Geometry: final body of the model. Coordinates: model frame, mm. Face numbers are marked on the shaded views. A direction names the side the tool comes from. Coordinates: 2 decimals unless noted, no trailing zeros. Write each loop counter-clockwise with the first axis right and the second up, starting at its lowest first coordinate (ties: lowest second). Pieces come first, ordered by that corner, then holes. Notation, with made-up numbers: (32.25, 46.5) -> (47.25, 46.5) arc R30 ccw to (47.25, 82.5) -> close; hole circle Ø7 at (84, -29.75). An arc over 180 degrees is marked (long way). One line per item, written item: value. Start each with the question number.
from build123d import *

# Parameters (mm, degrees)
SKETCH_1_R          = 1.5
EXTRUDE_1_DEPTH     = 23
SKETCH_2_R          = 1.5
EXTRUDE_2_DEPTH     = 8
SKETCH_3_R          = 2.4
SKETCH_3_R_2        = 1.5
EXTRUDE_3_DEPTH     = 0.5
CUT_EXTRUDE_START   = -1.5
SKETCH_4_R          = 1.5
SKETCH_4_R_2        = 1.25
CUT_EXTRUDE_1_DEPTH = 0.5


with BuildPart() as part:
    # 草图1 → 凸台-拉伸1 (new body)
    with BuildSketch(Plane(origin=(0, 0, 0), x_dir=(0, 0, -1), z_dir=(1, 0, 0))):
        Circle(SKETCH_1_R)
    extrude(amount=EXTRUDE_1_DEPTH)

    # 草图2 → 凸台-拉伸2 (add)
    with BuildSketch(Plane.ZY.offset(-9)):
        with BuildLine():
            Line((0.968245837, 1.75), (-0.968245837, 1.75))
            ThreePointArc((-0.968245837, 1.75), (0, -2), (0.968245837, 1.75))
        make_face()
        Circle(SKETCH_2_R, mode=Mode.SUBTRACT)
    extrude(amount=-EXTRUDE_2_DEPTH)

    # 草图3 → 凸台-拉伸3 (add)
    with BuildSketch(Plane(origin=(17, 0, 0), x_dir=(0, 0, -1), z_dir=(1, 0, 0))):
        Circle(SKETCH_3_R)
        with Locations(Location((0, 0, 0), (0, 0, 180))):
            Circle(SKETCH_3_R_2, mode=Mode.SUBTRACT)
    extrude(amount=EXTRUDE_3_DEPTH)

    # 草图4 → 切除-拉伸1 (cut)
    with BuildSketch(Plane(origin=(23, 0, 0), x_dir=(0, 0, -1), z_dir=(1, 0, 0)).offset(CUT_EXTRUDE_START)):
        Circle(SKETCH_4_R)
        Circle(SKETCH_4_R_2, mode=Mode.SUBTRACT)
    extrude(amount=CUT_EXTRUDE_1_DEPTH, mode=Mode.SUBTRACT)


solid = part.part
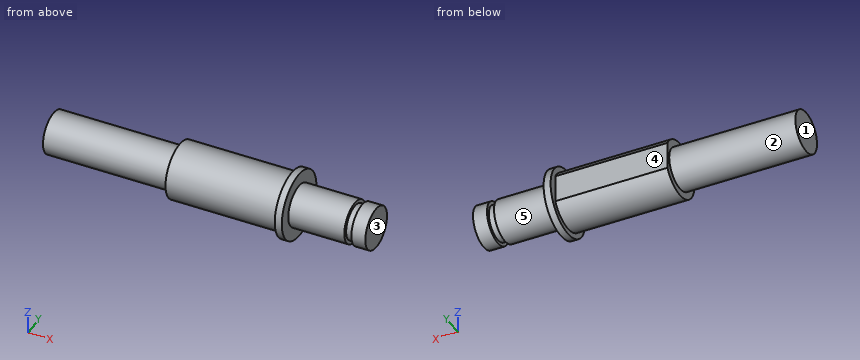
Q1. Cut plane B-B on y = 0. Output: boundary loops of the cut face in (x, z).
Q2. Cut plane D-D on x = 9.75. Output: boundary loops of the cut face in (y, z).
Q3. Line query: L1, parallel to X at y = 1.25, z = 0.55; L2, parallel to X at y = -1, z = 1.25; L3, parallel to X at y = 1.8, z = -0.05. Output: solid intervals per line, ascending. Write a range as from..to.
Q4. Access query for the marked faces 1, 2, 3, 4 and 5. Directions: +Z, -Z, +X, -X, +Y, -Y. A direction counts if a zero-diameter tool reaches every point of the face in a straight line with its end or side. Return the directions, or none.
Q5. Cut plane C-C on x = 3.25. Output: boundary loops of the cut face in (y, z), and give its area (3 significant figures).
Q6. Cut plane A-A on z = 0. Output: boundary loops of the cut face in (x, y).
Q7. First-contact query: P1, Ø0.6, axis at x = 11.5, z = 0, coming from the +Y side; P2, Ø1.5, axis at x = 9, y = 1, coming from the +Z side; P3, Ø1.5, axis at x = 7, y = 0.5, coming from the +Z side. Flat tips, straight axial feed; report the tip coordinate or a pass-through.
Solution:
1. outline: (0, -1.5) -> (9, -1.5) -> (9, -2) -> (17, -2) -> (17, -2.4) -> (17.5, -2.4) -> (17.5, -1.5) -> (21.5, -1.5) -> (21.5, -1.25) -> (22, -1.25) -> (22, -1.5) -> (23, -1.5) -> (23, 1.5) -> (22, 1.5) -> (22, 1.25) -> (21.5, 1.25) -> (21.5, 1.5) -> (17.5, 1.5) -> (17.5, 2.4) -> (17, 2.4) -> (17, 2) -> (9, 2) -> (9, 1.5) -> (0, 1.5) -> close
2. outline: (1.75, -0.97) -> (1.75, 0.97) arc R2 ccw (long way) to start
3. L1: 0..21.5, 22..23
3. L2: 9..17.5
3. L3: 17..17.5
4. face 1: +Z, -Z, -X, +Y, -Y
4. face 2: -X
4. face 3: +Z, -Z, +X, +Y, -Y
4. face 4: +Z, -Z, -X, +Y
4. face 5: +X
5. outline: circle Ø3 at (0, 0)
5. area: 7.07 mm²
6. outline: (0, -1.5) -> (9, -1.5) -> (9, -2) -> (17, -2) -> (17, -2.4) -> (17.5, -2.4) -> (17.5, -1.5) -> (21.5, -1.5) -> (21.5, -1.25) -> (22, -1.25) -> (22, -1.5) -> (23, -1.5) -> (23, 1.5) -> (22, 1.5) -> (22, 1.25) -> (21.5, 1.25) -> (21.5, 1.5) -> (17.5, 1.5) -> (17.5, 2.4) -> (17, 2.4) -> (17, 1.75) -> (9, 1.75) -> (9, 1.5) -> (0, 1.5) -> close
7. P1: y = 1.75
7. P2: z = 1.98
7. P3: z = 1.5
